Work out the finished part from the listing and answer in its coordinate system (mm). Face numbers are marked on the shaded views. Round coordinates to 2 decimals unless told otherwise and drop trailing zeros. Order: outer loops, then holes, each group sorted by start corner. A loop starts at its lowest first (then second) coordinate and runs counter-clockwise, first axis right, second up. Notation, with made-up numbers: (57.25, -25) -> (81.25, -25) arc R18 ccw to (81.25, -1) -> close; hole circle Ø11 at (19, -33). An arc over 180 degrees is marked (long way). Use a Markdown table: item, result. Add a question column.
Item 1: A cutting plane is placed at C-C, the plane x = 0. Determine the outline of the cut face in (y, z), plus the area to 3 significant figures.
Item 2: A cutting plane is placed at A-A, the plane z = 0. Determine the outline of the cut face in (x, y), plus the area to 3 significant figures.
Item 3: For a pull along Z with two mould halves and no side action, classify the marked faces 1, 2 and 3 as +Z half, -Z half, draft (parallel to the pull), parting line (faces both ways), or undercut.
Item 4: A cutting plane is placed at D-D, the plane z = 149. Determine the outline of the cut face in (x, y).
Item 5: Flat-ended cylindrical pins translate along their axes: P1, Ø8, axis at x = 31.5, z = -29, coming from the -Y side; P2, Ø5, axis at x = -127.5, y = 92.5, coming from the -Z side; P3, Ø6, axis at x = 114, z = 129.5, coming from the -Y side; P4, Ø10, axis at y = 216, z = -61.5, coming from the +X side. Find the tip coordinate at first contact, or state that the pin passes through.
Item 6: Find the intervals of material crossed by L1, parallel to X at y = 99, z = 0; L2, parallel to Y at x = -34, z = -55; L3, parallel to X at y = 296, z = 0, in increasing order. Write a range as [from, to].
Item 7: A cutting plane is placed at B-B, the plane x = 37.5. Determine the outline of the cut face in (y, z), plus the area to 3 significant figures.
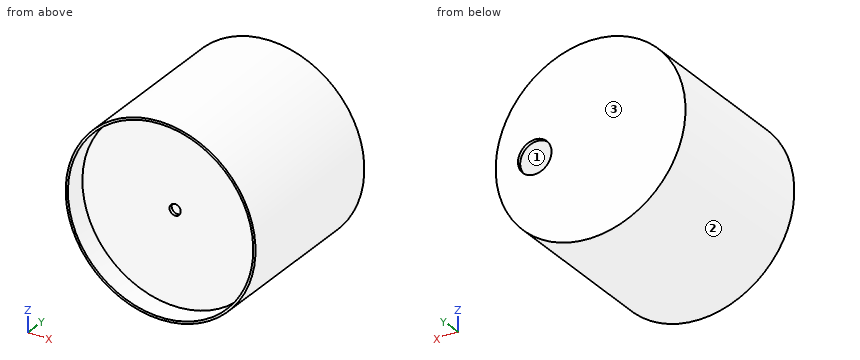
from build123d import *

# Parameters (mm, degrees)
RESERVOIR_WALL_SKETCH_R    = 170
RESERVOIR_WALL_SKETCH_R_2  = 166
RESERVOIR_WALL_SKIRT_DEPTH = 300
RESERVOIR_START            = 40
RESERVOIR_FLOOR_SKETCH_R   = 170
RESERVOIR_FLOOR_SKETCH_R_2 = 10
RESERVOIR_FLOOR_DEPTH      = 6
SEALED_START               = 294
SEALED_LID_SKETCH_R        = 170
SEALED_LID_SKETCH_R_2      = 30
SEALED_LID_DEPTH           = 6


with BuildPart() as part:
    # Reservoir Wall Sketch → Reservoir Wall + Skirt (new body)
    with BuildSketch(Plane(origin=(0, 0, 0), x_dir=(1, 0, 0), z_dir=(0, 1, 0))):
        with Locations(Location((0, 0, 0), (0, 0, 270))):
            Circle(RESERVOIR_WALL_SKETCH_R)
        with Locations(Location((0, 0, 0), (0, 0, 270))):
            Circle(RESERVOIR_WALL_SKETCH_R_2, mode=Mode.SUBTRACT)
    extrude(amount=RESERVOIR_WALL_SKIRT_DEPTH)

    # Reservoir Floor Sketch → Reservoir Floor (add)
    with BuildSketch(Plane(origin=(0, 0, 0), x_dir=(1, 0, 0), z_dir=(0, 1, 0)).offset(RESERVOIR_START)):
        with Locations(Location((0, 0, 0), (0, 0, 270))):
            Circle(RESERVOIR_FLOOR_SKETCH_R)
        with Locations(Location((0, 0, 0), (0, 0, 270))):
            Circle(RESERVOIR_FLOOR_SKETCH_R_2, mode=Mode.SUBTRACT)
    extrude(amount=RESERVOIR_FLOOR_DEPTH)

    # Sealed Lid Sketch → Sealed Lid (add)
    with BuildSketch(Plane(origin=(0, 0, 0), x_dir=(1, 0, 0), z_dir=(0, 1, 0)).offset(SEALED_START)):
        with Locations(Location((0, 0, 0), (0, 0, 270))):
            Circle(SEALED_LID_SKETCH_R)
        with Locations(Location((100, 0, 0), (0, 0, 270))):
            Circle(SEALED_LID_SKETCH_R_2, mode=Mode.SUBTRACT)
    extrude(amount=SEALED_LID_DEPTH)


solid = part.part
Reported:
| question | item | result |
|---|---|---|
| 1 | outline | (0, -170) -> (300, -170) -> (300, 170) -> (0, 170) -> (0, 166) -> (40, 166) -> (40, 10) -> (46, 10) -> (46, 166) -> (294, 166) -> (294, -166) -> (46, -166) -> (46, -10) -> (40, -10) -> (40, -166) -> (0, -166) -> close |
| 1 | area | 6,260 mm² |
| 2 | outline | (-170, 0) -> (-166, 0) -> (-166, 40) -> (-10, 40) -> (-10, 46) -> (-166, 46) -> (-166, 294) -> (70, 294) -> (70, 300) -> (-170, 300) -> close; (10, 40) -> (166, 40) -> (166, 0) -> (170, 0) -> (170, 300) -> (130, 300) -> (130, 294) -> (166, 294) -> (166, 46) -> (10, 46) -> close |
| 2 | area | 5,900 mm² |
| 3 | face 1 | undercut |
| 3 | face 2 | parting line |
| 3 | face 3 | draft |
| 4 | outline | (-81.85, 0) -> (-73.18, 0) -> (-73.18, 40) -> (73.18, 40) -> (73.18, 0) -> (81.85, 0) -> (81.85, 300) -> (-81.85, 300) -> close; hole (-73.18, 46) -> (73.18, 46) -> (73.18, 294) -> (-73.18, 294) -> close |
| 5 | P1 | y = 40 |
| 5 | P2 | z = -115.22 |
| 5 | P3 | y = 0 |
| 5 | P4 | x = 160.34 |
| 6 | L1 | [-170, -166], [166, 170] |
| 6 | L2 | [40, 46], [294, 300] |
| 6 | L3 | [-170, 70], [130, 170] |
| 7 | outline | (0, -165.81) -> (300, -165.81) -> (300, 165.81) -> (0, 165.81) -> (0, 161.71) -> (40, 161.71) -> (40, -161.71) -> (0, -161.71) -> close; hole (46, -161.71) -> (294, -161.71) -> (294, 161.71) -> (46, 161.71) -> close |
| 7 | area | 6,340 mm² |
